Verification items for the finished model (mm, model axes). Give positions to 0.01 mm unless a question says otherwise; leave off trailing zeros. Loops run counter-clockwise (first coordinate to the right, second up) from the corner with the lowest first, then second, coordinate; pieces in that order, holes last. Notation, with made-up numbers: (50, 36.5) - (56, 36.5) arc R28 cw to (56, 70.5) - close; hole circle Ø8 at (12.5, 44). An arc over 180 degrees is marked (long way). Use one line per item in the form item = value.
```python
from build123d import *

# Parameters (mm, degrees)
SKETCH_1_W          = 8
SKETCH_1_H          = 70
EXTRUDE_1_DEPTH     = 3
SKETCH_2_R          = 4
EXTRUDE_2_DEPTH     = 3
SKETCH_3_R          = 1.5
CUT_EXTRUDE_1_DEPTH = 3


with BuildPart() as part:
    # 草图1 → 凸台-拉伸1 (new body)
    with BuildSketch(Plane.XY):
        Rectangle(SKETCH_1_W, SKETCH_1_H)
    extrude(amount=EXTRUDE_1_DEPTH)

    # 草图2 → 凸台-拉伸2 (add)
    with BuildSketch(Plane.XY):
        with Locations((0, 35)):
            Circle(SKETCH_2_R)
        with Locations((0, -35)):
            Circle(SKETCH_2_R)
    extrude(amount=EXTRUDE_2_DEPTH)

    # 草图3 → 切除-拉伸1 (cut)
    with BuildSketch(Plane.XY.offset(3)):
        with Locations((0, 35)):
            Circle(SKETCH_3_R)
        with Locations((0, -35)):
            Circle(SKETCH_3_R)
    extrude(amount=-CUT_EXTRUDE_1_DEPTH, mode=Mode.SUBTRACT)


solid = part.part
```
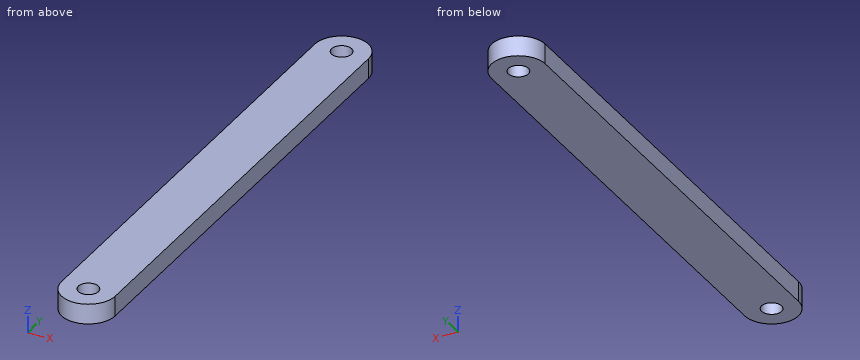
1. Section check A-A, the plane x = 0. Record the cut outline in (y, z), then the cut area to 3 significant figures.
Result set:
outline = (-39, 0) - (-36.5, 0) - (-36.5, 3) - (-39, 3) - close; (-33.5, 0) - (33.5, 0) - (33.5, 3) - (-33.5, 3) - close; (36.5, 0) - (39, 0) - (39, 3) - (36.5, 3) - close
area = 216 mm²
2. Depth check by flat-ended pin: pin 1 Ø1.8 at (x, y) = (0, 35) entering from +Z (1 decimal); pin 2 Ø1 at (x, z) = (-2, 1) entering from -Y. Enter the tip coordinate at first touch or a pass-through.
Result set:
pin_1 = through
pin_2 = -38.71
3. Scan lines: probe 1 along Y at (x, z) = (0, 1.95); probe 2 along Y at (x, z) = (-1, 2.15); probe 3 along Y at (x, z) = (-2.5, 1.8). Record each from-to range of solid material in increasing order.
Result set:
probe_1 = -39 to -36.5, -33.5 to 33.5, 36.5 to 39
probe_2 = -38.87 to -36.12, -33.88 to 33.88, 36.12 to 38.87
probe_3 = -38.12 to 38.12
4. Section check B-B, the plane z = 0.9. Record the cut outline in (x, y).
Result set:
outline = (-4, -35) arc R4 ccw to (4, -35) - (4, 35) arc R4 ccw to (-4, 35) - close; hole circle Ø3 at (0, -35); hole circle Ø3 at (0, 35)
5. Section check C-C, the plane x = -2.75. Record the cut outline in (y, z), then the cut area to 3 significant figures.
Result set:
outline = (-37.9, 0) - (37.9, 0) - (37.9, 3) - (-37.9, 3) - close
area = 227 mm²
